from build123d import *

# Parameters (mm, degrees)
SKETCH1_R           = 1.5
BOSS_EXTRUDE1_DEPTH = 5
SKETCH2_W           = 2.494401268
SKETCH2_H           = 15.1
BOSS_EXTRUDE2_DEPTH = 1
SKETCH3_W           = 13
SKETCH3_H           = 1.3
CUT_EXTRUDE1_DEPTH  = 21.029562163
SKETCH4_W           = 2
SKETCH4_H           = 0.923045376
SKETCH4_H_2         = 1
BOSS_EXTRUDE3_DEPTH = 1.14
SKETCH5_W           = 2
SKETCH5_H           = 8.923045376
BOSS_EXTRUDE4_DEPTH = 1
FILLET1_R           = 1
FILLET2_R           = 0.5


with BuildPart() as part:
    # Sketch1 → Boss-Extrude1 (new body)
    with BuildSketch(Plane(origin=(0, 0, 0), x_dir=(1, 0, 0), z_dir=(0, 1, 0))):
        Polygon((5.958367707, 12.55), (-5.958367707, 12.55), (-8.452768975, 12.55), (-8.452768975, -12.55), (-5.958367707, -12.55), (5.958367707, -12.55), (5.958367707, -7.55), (-5.958367707, -7.55), (-5.958367707, 7.55), (5.958367707, 7.55), align=None)
        with Locations(Location((-3.458367707, -10.05, 0), (0, 0, 270))):
            Circle(SKETCH1_R, mode=Mode.SUBTRACT)
        with Locations(Location((-3.458367707, 10.05, 0), (0, 0, 90))):
            Circle(SKETCH1_R, mode=Mode.SUBTRACT)
    extrude(amount=BOSS_EXTRUDE1_DEPTH)

    # Sketch2 → Boss-Extrude2 (add)
    with BuildSketch(Plane(origin=(0, 5, 0), x_dir=(1, 0, 0), z_dir=(0, 1, 0))):
        with Locations((-7.205568341, 0)):
            Rectangle(SKETCH2_W, SKETCH2_H)
    extrude(amount=BOSS_EXTRUDE2_DEPTH)

    # Sketch3 → Cut-Extrude1 (cut, through all)
    with BuildSketch(Plane.ZY.offset(8.452768975)):
        with Locations((0, 0.65)):
            Rectangle(SKETCH3_W, SKETCH3_H)
    extrude(amount=-CUT_EXTRUDE1_DEPTH, mode=Mode.SUBTRACT)

    # Sketch4 → Boss-Extrude3 (add)
    with BuildSketch(Plane(origin=(0, 6, 0), x_dir=(1, 0, 0), z_dir=(0, 1, 0))):
        with Locations((-7.205568341, -4.461522688)):
            Rectangle(SKETCH4_W, SKETCH4_H)
        with Locations((-7.205568341, 3.5)):
            Rectangle(SKETCH4_W, SKETCH4_H_2)
    extrude(amount=BOSS_EXTRUDE3_DEPTH)

    # Sketch5 → Boss-Extrude4 (add)
    with BuildSketch(Plane(origin=(0, 7.14, 0), x_dir=(1, 0, 0), z_dir=(0, 1, 0))):
        with Locations((-7.205568341, -0.461522688)):
            Rectangle(SKETCH5_W, SKETCH5_H)
    extrude(amount=BOSS_EXTRUDE4_DEPTH)

    # Fillet1
    fillet1_edges = [part.edges().sort_by_distance(p)[0] for p in [
        (5.958367707, 2.5, -7.55),
        (5.958367707, 2.5, 7.55),
        (5.958367707, 2.5, 12.55),
        (-8.452768975, 2.5, 12.55),
        (-8.452768975, 2.5, -12.55),
        (5.958367707, 2.5, -12.55),
    ]]
    fillet(fillet1_edges, radius=FILLET1_R)

    # Fillet2
    fillet2_edges = [part.edges().sort_by_distance(p)[0] for p in [
        (-5.958367707, 5.5, 7.55),
        (-5.958367707, 5.5, -7.55),
        (-8.452768975, 5.5, -7.55),
        (-8.452768975, 5.5, 7.55),
        (-8.205568341, 7.07, 4.923045376),
        (-6.205568341, 7.07, 4.923045376),
        (-6.205568341, 7.07, -4),
        (-8.205568341, 7.07, -4),
    ]]
    fillet(fillet2_edges, radius=FILLET2_R)


solid = part.part
Geometry check sheet. Reference: the model listing, model coordinates, mm. A direction names the side the tool comes from. Give positions to 0.01 mm unless a question says otherwise; leave off trailing zeros. Loops run counter-clockwise (first coordinate to the right, second up) from the corner with the lowest first, then second, coordinate; pieces in that order, holes last.
(1) Depth check by flat-ended pin: pin 1 Ø2 at (x, z) = (0, 6) entering from +Y; pin 2 Ø0.5 at (x, y) = (-7, 5.5) entering from -Z; pin 3 Ø0.6 at (x, y) = (-7, 7) entering from -Z; pin 4 Ø3 at (x, z) = (2, 11) entering from +Y. Enter the tip coordinate at first touch or a pass-through.
From the geometry:
pin 1: passes through
pin 2: stops at z = -7.55
pin 3: stops at z = -4
pin 4: stops at y = 5
(2) Section check D-D on y = 0.5. Record the cut outline in (x, z).
From the geometry:
outline: (-8.45, -11.55) arc R1 ccw to (-7.45, -12.55) - (4.96, -12.55) arc R1 ccw to (5.96, -11.55) - (5.96, -8.55) arc R1 ccw to (4.96, -7.55) - (-5.96, -7.55) - (-5.96, -6.5) - (-8.45, -6.5) - close; (-8.45, 6.5) - (-5.96, 6.5) - (-5.96, 7.55) - (4.96, 7.55) arc R1 ccw to (5.96, 8.55) - (5.96, 11.55) arc R1 ccw to (4.96, 12.55) - (-7.45, 12.55) arc R1 ccw to (-8.45, 11.55) - close; hole circle Ø3 at (-3.46, -10.05); hole circle Ø3 at (-3.46, 10.05)
(3) Set-up check for faces 5 (the flat face through (-7.2, 5.5, 7.55)), 6 (the flat face through (-7, 1.3, 0)), 7 (the flat face through (-5.958, 4, 0)): record each of +Z, -Z, +X, -X, +Y, -Y from which the full face is reachable in a straight line by a thin tool's end or side.
From the geometry:
face 5: +Z, +X, -X, +Y
face 6: +X, -X, -Y
face 7: +X, +Y, -Y
(4) Release check for a two-part mould opening along Z. For faces 1 (the flat face through (-7, 8.14, 0)), 2 (the flat face through (-1, 2, 12.55)), 3 (the cylindrical face through (5.66, 2.54, -12.26)), 4 (the flat face through (-7.2, 6.6, 4)) record: released by +Z, released by -Z, zero draft, split by the parting line, or undercut.
From the geometry:
face 1: zero draft
face 2: released by +Z
face 3: released by -Z
face 4: undercut
(5) Thickness scan on L1, parallel to Z at x = -4.25, y = 2.5; L2, parallel to Z at x = 4.5, y = 4.5; L3, parallel to X at y = 1.85, z = -10.05. Record the ranges inside material, lowest first.
From the geometry:
L1: z = -12.55 to -11.32, -8.78 to -7.55, 7.55 to 8.78, 11.32 to 12.55
L2: z = -12.55 to -7.55, 7.55 to 12.55
L3: x = -8.45 to -4.96, -1.96 to 5.96
(6) Section check B-B on z = -10.05. Record the cut outline in (x, y), then the cut area to 3 significant figures.
From the geometry:
outline: (-8.45, 0) - (-4.96, 0) - (-4.96, 5) - (-8.45, 5) - close; (-1.96, 0) - (5.96, 0) - (5.96, 5) - (-1.96, 5) - close
area: 57.1 mm2
(7) Section check C-C on y = 6.25. Record the cut outline in (x, z).
From the geometry:
outline: (-8.21, -3.5) arc R0.5 ccw to (-7.71, -4) - (-6.71, -4) arc R0.5 ccw to (-6.21, -3.5) - (-6.21, -3) - (-8.21, -3) - close; (-8.21, 4) - (-6.21, 4) - (-6.21, 4.42) arc R0.5 ccw to (-6.71, 4.92) - (-7.71, 4.92) arc R0.5 ccw to (-8.21, 4.42) - close
(8) Section check A-A on x = -1. Record the cut outline in (y, z), then the cut area to 3 significant figures.
From the geometry:
outline: (0, -12.55) - (5, -12.55) - (5, -7.55) - (0, -7.55) - close; (0, 7.55) - (5, 7.55) - (5, 12.55) - (0, 12.55) - close
area: 50.0 mm2
